Design review of the part built by this model. Coordinates are the model's own, in mm. A direction names the side the tool comes from. Coordinates: 2 decimals unless noted, no trailing zeros. Loops run counter-clockwise (first coordinate to the right, second up) from the corner with the lowest first, then second, coordinate; pieces in that order, holes last.
Q1. Draft analysis for pull direction X (two halves, no side actions). For faces 3 (the face through (54, -26.5, 0)), 4 (the face through (71.7, -29, -13.6)), state which applies: released by +X, released by -X, zero draft, split by the parting line, or undercut.
Q2. Add section D-D on z = -9.5. Give the boundary of the cut face in (x, y).
Q3. Wall thickness on probe 1 along X at (y, z) = (-12, 0); probe 2 along X at (y, z) = (4, 0); probe 3 along Y at (x, z) = (67, -12): over which ranges is each line inside the solid? List them lowest first.
Q4. Machinability: for faces 1 (the face through (-9.1, 0, -22.1)), 2 (the face through (71.7, -29.04, 14.68)), which of the approach directions +Z, -Z, +X, -X, +Y, -Y give a long, thin tool a straight path to every point of the face, cutting with its end or side? Answer none if there is none.
Q5. Add section B-B on x = 75.5. Give the boundary of the cut face in (y, z).
Q6. For P1, Ø4.5, axis at x = 45.86, z = -14.14, coming from the -Y side; P2, Ø8, axis at x = 74.14, z = -14.14, coming from the +Y side; P3, Ø8, axis at x = 13, y = -1, coming from the +Z side; P4, Ø10, axis at y = -11, z = -17, coming from the +X side, all flat-tipped, find the tip position at first contact; note any pin that passes through.
Q7. Add section A-A on z = 0. Give the boundary of the cut face in (x, y), and give its area (3 significant figures).
Q8. Add section C-C on x = -10. Give the boundary of the cut face in (y, z).
```python
from build123d import *

# Parameters (mm, degrees)
SKETCH1_R           = 26
SKETCH1_R_2         = 24.95
BOSS_EXTRUDE1_DEPTH = 7.5
BOSS_EXTRUDE2_START = 31.5
SKETCH2_R           = 26
SKETCH2_R_2         = 23.75
BOSS_EXTRUDE2_DEPTH = 31.5
SKETCH3_R           = 23.75
BOSS_EXTRUDE3_DEPTH = 1
SKETCH4_R           = 3
CUT_EXTRUDE1_DEPTH  = 1
BOSS_EXTRUDE4_DEPTH = 5
SKETCH6_R           = 2.5
CUT_EXTRUDE2_DEPTH  = 5


with BuildPart() as part:
    # Sketch1 → Boss-Extrude1 (new body)
    with BuildSketch(Plane(origin=(0, 0, 0), x_dir=(1, 0, 0), z_dir=(0, 1, 0))):
        with Locations(Location((0, 0, 0), (0, 0, 270))):
            Circle(SKETCH1_R)
        with Locations(Location((0, 0, 0), (0, 0, 270))):
            Circle(SKETCH1_R_2, mode=Mode.SUBTRACT)
    extrude(amount=BOSS_EXTRUDE1_DEPTH)

    # Sketch2 → Boss-Extrude2 (add)
    with BuildSketch(Plane.XZ.offset(BOSS_EXTRUDE2_START)):
        with Locations(Location((0, 0, 0), (0, 0, 270))):
            Circle(SKETCH2_R)
        with Locations(Location((0, 0, 0), (0, 0, 270))):
            Circle(SKETCH2_R_2, mode=Mode.SUBTRACT)
    extrude(amount=-BOSS_EXTRUDE2_DEPTH)

    # Sketch3 → Boss-Extrude3 (add)
    with BuildSketch(Plane.XZ.offset(31.5)):
        with Locations(Location((0, 0, 0), (0, 0, 270))):
            Circle(SKETCH3_R)
    extrude(amount=-BOSS_EXTRUDE3_DEPTH)

    # Sketch4 → Cut-Extrude1 (cut)
    with BuildSketch(Plane.XZ.offset(31.5)):
        with Locations(Location((0, 0, 0), (0, 0, 270))):
            Circle(SKETCH4_R)
    extrude(amount=-CUT_EXTRUDE1_DEPTH, mode=Mode.SUBTRACT)

    # Sketch5 → Boss-Extrude4 (add)
    with BuildSketch(Plane.XZ.offset(31.5)):
        with BuildLine():
            Line((-0.468, 25.995787659), (59.51256, 27.075612685))
            ThreePointArc((59.51256, 27.075612685), (87.08, 0), (59.51256, -27.075612685))
            Line((59.51256, -27.075612685), (-0.468, -25.995787659))
            ThreePointArc((-0.468, -25.995787659), (26, 0), (-0.468, 25.995787659))
        make_face()
    extrude(amount=-BOSS_EXTRUDE4_DEPTH)

    # Sketch6 → Cut-Extrude2 (cut)
    with BuildSketch(Plane.XZ.offset(31.5)):
        with Locations(Location((74.142135624, 14.142135624, 0), (0, 0, 270))):
            Circle(SKETCH6_R)
        with Locations(Location((74.142135624, -14.142135624, 0), (0, 0, 270))):
            Circle(SKETCH6_R)
        with Locations(Location((45.857864376, -14.142135624, 0), (0, 0, 270))):
            Circle(SKETCH6_R)
        with Locations(Location((45.857864376, 14.142135624, 0), (0, 0, 270))):
            Circle(SKETCH6_R)
    extrude(amount=-CUT_EXTRUDE2_DEPTH, mode=Mode.SUBTRACT)


solid = part.part
```
Entries:
1. face 3: zero draft
1. face 4: undercut
2. outline: (-24.2, -31.5) - (85.36, -31.5) - (85.36, -26.5) - (24.2, -26.5) - (24.2, 7.5) - (23.07, 7.5) - (23.07, 0) - (21.77, 0) - (21.77, -30.5) - (-21.77, -30.5) - (-21.77, 0) - (-23.07, 0) - (-23.07, 7.5) - (-24.2, 7.5) - close
3. probe 1: x = -26 to -23.75, 23.75 to 26
3. probe 2: x = -26 to -24.95, 24.95 to 26
3. probe 3: y = -31.5 to -26.5
4. face 1: +Y
4. face 2: +Y, -Y
5. outline: (-31.5, -22.21) - (-26.5, -22.21) - (-26.5, -16.24) - (-31.5, -16.24) - close; (-31.5, -12.04) - (-26.5, -12.04) - (-26.5, 12.04) - (-31.5, 12.04) - close; (-31.5, 16.24) - (-26.5, 16.24) - (-26.5, 22.21) - (-31.5, 22.21) - close
6. P1: passes through
6. P2: stops at y = -26.5
6. P3: stops at z = 24.39
6. P4: stops at x = 23.07
7. outline: (-26, -31.5) - (-3, -31.5) - (-3, -30.5) - (-23.75, -30.5) - (-23.75, 0) - (-24.95, 0) - (-24.95, 7.5) - (-26, 7.5) - close; (3, -31.5) - (87.08, -31.5) - (87.08, -26.5) - (26, -26.5) - (26, 7.5) - (24.95, 7.5) - (24.95, 0) - (23.75, 0) - (23.75, -30.5) - (3, -30.5) - close
7. area: 504 mm2
8. outline: (-31.5, -24) - (7.5, -24) - (7.5, -22.86) - (0, -22.86) - (0, -21.54) - (-30.5, -21.54) - (-30.5, 21.54) - (0, 21.54) - (0, 22.86) - (7.5, 22.86) - (7.5, 24) - (-31.5, 24) - close
